from build123d import *

# Parameters (mm, degrees)
F4_T = -0.5


with BuildPart() as f3:
    # F0 (on Top) → F3 section 0
    with BuildSketch(Plane.XY):
        with BuildLine():
            ThreePointArc((-87.5, -52), (-85.156854, -57.656854), (-79.5, -60))
            Line((-79.5, -60), (79.5, -60))
            ThreePointArc((79.5, -60), (85.156854, -57.656854), (87.5, -52))
            Line((87.5, -52), (87.5, 52))
            ThreePointArc((87.5, 52), (85.156854, 57.656854), (79.5, 60))
            Line((79.5, 60), (-79.5, 60))
            ThreePointArc((-79.5, 60), (-85.156854, 57.656854), (-87.5, 52))
            Line((-87.5, 52), (-87.5, -52))
        make_face()
    # F2 (on offset) → F3 section 1
    with BuildSketch(Plane.XY.offset(60)):
        with BuildLine():
            Line((67.5, 45), (-67.5, 45))
            ThreePointArc((-67.5, 45), (-71.035534, 43.535534), (-72.5, 40))
            Line((-72.5, 40), (-72.5, -40))
            ThreePointArc((-72.5, -40), (-71.035534, -43.535534), (-67.5, -45))
            Line((-67.5, -45), (67.5, -45))
            ThreePointArc((67.5, -45), (71.035534, -43.535534), (72.5, -40))
            Line((72.5, -40), (72.5, 40))
            ThreePointArc((72.5, 40), (71.035534, 43.535534), (67.5, 45))
        make_face()
    loft()

    # F4
    f4_openings = [f3.faces().sort_by_distance(p)[0] for p in [
        (0, 0, 0),
    ]]
    offset(amount=F4_T, openings=f4_openings)


solid = f3.part
Check sheet for the modelled part. Datum: model origin and axes. Units: mm. Round coordinates to 2 decimals unless told otherwise and drop trailing zeros. One line per item, written item: value. Start each with the question number.
1. Gauge pin test, flat ends, axial feed: P1, Ø2, axis at y = 29.5, z = 28.5, coming from the -X side (3 decimals); P2, Ø5, axis at x = 30.5, z = 46.5, coming from the -Y side; P3, Ø4, axis at x = 46.5, z = 48, coming from the -Y side. Record the tip position at first contact, or that the pin passes through.
2. Release check for a two-part mould opening along X. For faces 1 (the flat face through (-1.113, -51.943, 30.166)), 2 (the flat face through (1, -1, 60)), 3 (the flat face through (79.443, -0.728, 30.166)) record: released by +X, released by -X, zero draft, split by the parting line, or undercut.
3. Scan lines: line 1 along Z through (x, y) = (-45, 10); line 2 along X through (y, z) = (-49.5, 34); line 3 along X through (y, z) = (-2, 33.5) (3 decimals). Record each from-to range of solid material in increasing order.
Results found:
1. P1: x = -80.625
1. P2: y = -49
1. P3: y = -48.5
2. face 1: undercut
2. face 2: zero draft
2. face 3: undercut
3. line 1: 59.5 to 60
3. line 2: -77.3 to -76.55, 76.55 to 77.3
3. line 3: -79.125 to -78.61, 78.61 to 79.125
